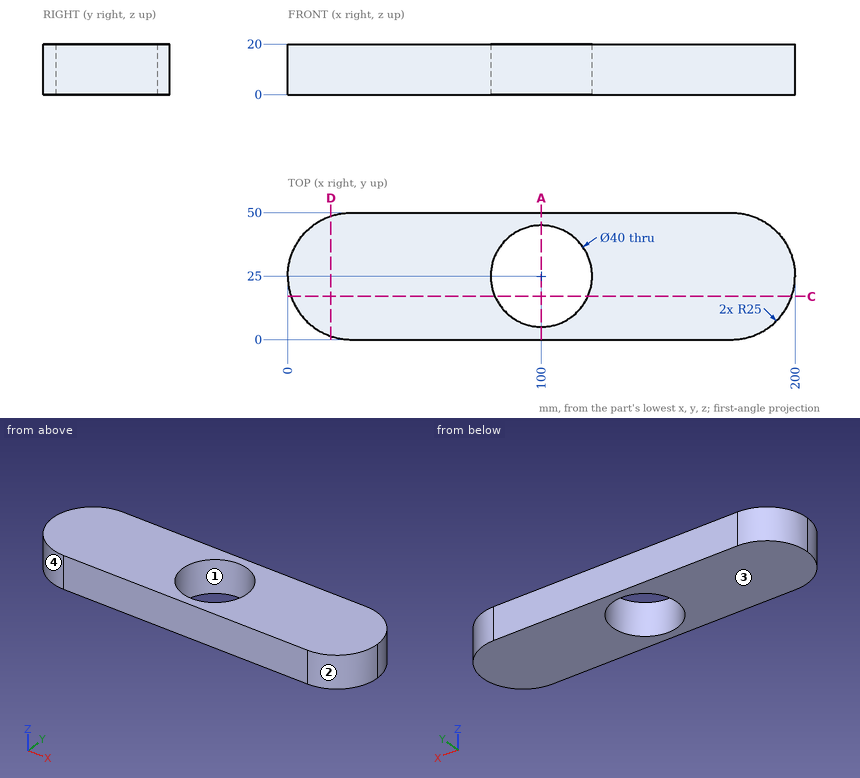
Design review of the part shown in the three views and the two pictorial views. Dimensions are in mm from the part's minimum x, y and z. Round coordinates to 2 decimals unless told otherwise and drop trailing zeros. Order: outer loops, then holes, each group sorted by start corner. A loop starts at its lowest first (then second) coordinate and runs counter-clockwise, first axis right, second up. Notation, with made-up numbers: (5, -6.5) -> (39, -6.5) arc R8 cw to (39, 8.5) -> close; hole circle Ø8 at (16.25, -32). An arc over 180 degrees is marked (long way). Write item = value, one per line. Start each with the question number.
1) Insertion check: pin 1 (24 mm diameter, centred on x = 100, y = 25, fed in from -Z); pin 2 (3 mm diameter, centred on y = 37.5, z = 15.5, fed in from -X). Each pin has a flat end and moves straight along its axis. Give the tip position at first contact, or say it passes through.
2) To check wall thickness, follow line 1 (Y direction, x = 100, z = 16.25); line 2 (Y direction, x = 84.5, z = 10.25); line 3 (X direction, y = 15, z = 4.5). State the ranges of each line that lie inside material, in increasing order. Write a range as from..to.
3) Take a section at C-C on y = 17. State the section outline as (x, z) points, plus the area to 3 significant figures.
4) Take a section at D-D on x = 17. State the section outline as (y, z) points.
5) Take a section at A-A on x = 100. State the section outline as (y, z) points, plus the area to 3 significant figures.
6) The part is to be moulded in two halves that separate along X. For the marked faces 1, 2, 3 and 4, say which applies: +X half, -X half, draft (parallel to the pull), parting line (faces both ways), or undercut.
Verdict:
q1.pin_1 = through
q1.pin_2 = 2.55
q2.line_1 = 0..5, 45..50
q2.line_2 = 0..12.36, 37.64..50
q2.line_3 = 2.09..82.68, 117.32..197.91
q3.outline = (1.31, 0) -> (81.67, 0) -> (81.67, 20) -> (1.31, 20) -> close; (118.33, 0) -> (198.69, 0) -> (198.69, 20) -> (118.33, 20) -> close
q3.area = 3,210 mm2
q4.outline = (1.31, 0) -> (48.69, 0) -> (48.69, 20) -> (1.31, 20) -> close
q5.outline = (0, 0) -> (5, 0) -> (5, 20) -> (0, 20) -> close; (45, 0) -> (50, 0) -> (50, 20) -> (45, 20) -> close
q5.area = 200 mm2
q6.face_1 = undercut
q6.face_2 = +X half
q6.face_3 = draft
q6.face_4 = -X half
